Could you check a few things on this model? Use its own coordinates, in mm. A direction names the side the tool comes from. Round coordinates to 2 decimals unless told otherwise and drop trailing zeros. Write each loop counter-clockwise with the first axis right and the second up, starting at its lowest first coordinate (ties: lowest second). Pieces come first, ordered by that corner, then holes. Notation, with made-up numbers: (58.5, 30.5) -> (102.5, 30.5) arc R26 ccw to (102.5, 54.5) -> close; hole circle Ø11 at (45.5, -20.5). An arc over 180 degrees is marked (long way). Answer as CSV lines item,"result". Start each with the question number.
Q1. Imagine slicing it at B-B on x = 114.3. Please give me the cut outline in (y, z).
Q2. If I drill on line 1 (X direction, y = 152, z = 1); line 2 (Y direction, x = 60, z = 23.5), over which ranges is the centre line in solid material (lowest first)? Write a range as [from, to].
Q3. Will these pins go through, and if not, where does the flat tip stop? pin 1 Ø5.5 at (x, y) = (118.85, 124.1) entering from +Z; pin 2 Ø8 at (x, y) = (37, 85.5) entering from -Z; pin 3 Ø9.5 at (x, z) = (65.5, 28.5) entering from +Y; pin 4 Ø3.5 at (x, y) = (21.44, 152.4) entering from +Z.
Q4. Imagine slicing it at C-C on z = 13.5. Please give me the cut outline in (x, y).
Q5. For faces 4 (the flat face through (69, 106, 0)), 5 (the flat face through (71, 3.048, 22)), which set-ups out of +Z, -Z, +X, -X, +Y, -Y let a thin tool reach every point of the face, with its end or its side?
Q6. Imagine slicing it at A-A on y = 152.4. Please give me the cut outline in (x, z).
Q7. Imagine slicing it at D-D on x = 69.85. Please give me the cut outline in (y, z), and give its area (3 significant figures).
Q8. If we mould it in two halves opening along Y, with no side actions, what happens to faces 1 (the flat face through (0, 101, 2)), 2 (the cylindrical face through (69.01, 171.43, 1.5)), 3 (the cylindrical face through (70.83, 1.74, 1.83))? For each: pulls with the +Y half, pulls with the -Y half, needs draft (parallel to the pull), parting line crosses it, or undercut.
Autodesk Inventor part; units mm, degrees
ref_plane "YZ Plane" through (0, 0, 0) normal (1, 0, 0) x (0, 1, 0)
ref_plane "XZ Plane" through (0, 0, 0) normal (0, 1, 0) x (-1, 0, 0)
ref_plane "XY Plane" through (0, 0, 0) normal (0, 0, 1) x (1, 0, 0)
sketch "Sketch1" plane through (0, 0, 0) normal (0, 0, 1) x (1, 0, 0)
  line L0 (0, 0) -> (139.7, 0)
  line L1 (139.7, 0) -> (139.7, 203.2)
  line L2 (139.7, 203.2) -> (0, 203.2)
  line L3 (0, 203.2) -> (0, 0)
  dimension "d0" = 139.7
  dimension "d1" = 203.2
extrude "Plate1" add sketch "Sketch1" along normal blind 3.048
sketch "Sketch2" plane through (139.7, 3.048, 0) normal (0, -1, 0) x (1, 0, 0)
  line L0 (-139.7, 0) -> (0, 0)
  line L1 (0, 0) -> (0, 38.1)
  line L2 (0, 38.1) -> (-139.7, 38.1)
  line L3 (-139.7, 38.1) -> (-139.7, 0)
edge flange "Flange1" height 38.1 angle 90 thickness 3.048 bend radius 3.048 thickness toward (0, -1, 0) relief tear relief width 3.048 relief depth 1.524 edges at (69.85, 0, 3.048) wall of the first edge with corners at (0, 3.048, 0) (139.7, 3.048, 0) (139.7, 3.048, 38.1) (0, 3.048, 38.1)
bend "Bend1"
corner "Corner1"
sketch "Sketch3" plane through (0, 0, 3.048) normal (0, 0, 1) x (1, 0, 0)
  line L0 (139.7, 203.2) -> (139.7, 6.096)
  line L1 (0, 203.2) -> (139.7, 203.2)
  circle A0 centre (21.4376, 152.4) radius 2.0638
  circle A1 centre (118.8466, 124.1044) radius 2.0638
  circle A2 centre (118.6688, 180.9242) radius 2.0637
  point P0 (0, 0)
  dimension "d13" = 20.8534
  dimension "d14" = 79.0956
  dimension "d16" = 21.0312
  dimension "d18" = 50.8
  dimension "d19" = 22.2758
  dimension "d20" = 4.1275
  dimension "d21" = 4.1275
  dimension "d22" = 4.1275
  dimension "d39" = 118.2624
hole "Hole1" at (118.8466, 124.1044, 3.048) at (118.6688, 180.9242, 3.048) at (21.4376, 152.4, 3.048) direction (0, 0, -1) diameter 4.1275 end through all
sketch "Sketch4" plane through (0, 3.048, 38.1) normal (0, 1, 0) x (1, 0, 0)
  line L0 (0, 0) -> (0, 32.004)
  line L1 (139.7, 0) -> (139.7, 32.004)
  point P0 (0, 38.1)
  point P1 (25.4, 16.002)
  point P2 (114.3, 16.002)
  dimension "d30" = 25.4
  dimension "d31" = 25.4
hole "Hole2" at (25.4, 3.048, 22.098) at (114.3, 3.048, 22.098) direction (0, -1, 0) diameter 6.35 end through all
sketch "Sketch5" plane through (0, 0, 3.048) normal (0, 0, 1) x (1, 0, 0)
  line L0 (139.7, 203.2) -> (139.7, 6.096)
  line L1 (0, 203.2) -> (139.7, 203.2)
  point P0 (0, 0)
  point P1 (69.85, 152.4)
  dimension "d40" = 50.8
  dimension "d41" = 69.85
hole "Hole3" at (69.85, 152.4, 3.048) direction (0, 0, -1) diameter 38.1 end through all
equation "\"d28\" = Thickness"
equation "\"d37\" = Thickness"
equation "\"d47\" = Thickness"
equation "\"d3\" = BendReliefWidth"
equation "\"d4\" = BendReliefDepth"
equation "\"d5\" = MinimumRemnant"
equation "\"d6\" = BendRadius"
equation "\"d9\" = BendRadius"
equation "\"d10\" = CornerReliefSize"
equation "\"d11\" = GapSize"
equation "\"d12\" = JacobiRadiusSize"
equation "\"BendRadius\" = Thickness"
equation "\"BendReliefWidth\" = Thickness"
equation "\"BendReliefDepth\" = 0.5 * Thickness"
equation "\"CornerReliefSize\" = 4 * Thickness"
equation "\"MinimumRemnant\" = 2 * Thickness"
equation "\"TransitionRadius\" = BendRadius"
equation "\"JacobiRadiusSize\" = BendRadius"
equation "\"GapSize\" = Thickness"
equation "\"d2\" = BendRadius"
properties material "Aluminum 6061"
Checks:
1,outline,"(0, 6.1) arc R6.1 ccw to (6.1, 0) -> (203.2, 0) -> (203.2, 3.05) -> (6.1, 3.05) arc R3.05 cw to (3.05, 6.1) -> (3.05, 18.92) -> (0, 18.92) -> close; (0, 25.27) -> (3.05, 25.27) -> (3.05, 38.1) -> (0, 38.1) -> close"
2,line 1,"[0, 19.41], [23.46, 50.8], [88.9, 139.7]"
2,line 2,"[0, 3.05]"
3,pin 1,"z = 3.05"
3,pin 2,"z = 0"
3,pin 3,"y = 3.05"
3,pin 4,"through"
4,outline,"(0, 0) -> (139.7, 0) -> (139.7, 3.05) -> (0, 3.05) -> close"
5,face 4,"-Z, +X, -X, +Y, -Y"
5,face 5,"+Z, +X, -X, +Y"
6,outline,"(0, 0) -> (19.37, 0) -> (19.37, 3.05) -> (0, 3.05) -> close; (23.5, 0) -> (50.8, 0) -> (50.8, 3.05) -> (23.5, 3.05) -> close; (88.9, 0) -> (139.7, 0) -> (139.7, 3.05) -> (88.9, 3.05) -> close"
7,outline,"(0, 6.1) arc R6.1 ccw to (6.1, 0) -> (133.35, 0) -> (133.35, 3.05) -> (6.1, 3.05) arc R3.05 cw to (3.05, 6.1) -> (3.05, 38.1) -> (0, 38.1) -> close; (171.45, 0) -> (203.2, 0) -> (203.2, 3.05) -> (171.45, 3.05) -> close"
7,area,"604 mm^2"
8,face 1,"needs draft"
8,face 2,"undercut"
8,face 3,"pulls with the -Y half"
